from build123d import *

# Parameters (mm, degrees)
SKETCH_1_R                      = 75
SKETCH_1_R_2                    = 50
EXTRUDE_1_DEPTH                 = 50
SKETCH_2_R                      = 525
SKETCH_2_R_2                    = 500
EXTRUDE_2_DEPTH                 = 50
EXTRUDE_4_DEPTH                 = 25
CUT_EXTRUDE_1_DEPTH             = 10
PATTERN_CIRCULAR_1_COUNT        = 5
PATTERN_CIRCULAR_1_COPY_1_DEPTH = 10
PATTERN_CIRCULAR_1_COPY_2_DEPTH = 10
PATTERN_CIRCULAR_1_COPY_3_DEPTH = 10
PATTERN_CIRCULAR_1_COPY_4_DEPTH = 10


with BuildPart() as part:
    # Sketch 1 → Extrude 1 (new body, symmetric)
    with BuildSketch(Plane(origin=(0, 0, 0), x_dir=(1, 0, 0), z_dir=(0, 1, 0))):
        Circle(SKETCH_1_R)
        Circle(SKETCH_1_R_2, mode=Mode.SUBTRACT)
    extrude(amount=EXTRUDE_1_DEPTH, both=True)



with BuildPart() as body_2:
    # Sketch 2 → Extrude 2 (new body, symmetric)
    with BuildSketch(Plane(origin=(0, 0, 0), x_dir=(1, 0, 0), z_dir=(0, 1, 0))):
        Circle(SKETCH_2_R)
        Circle(SKETCH_2_R_2, mode=Mode.SUBTRACT)
    extrude(amount=EXTRUDE_2_DEPTH, both=True)


with BuildPart() as part_1:
    add(part.part)

    add(body_2.part)  # Extrude 4 merges body 2
    # Sketch 3 → Extrude 4 (add, symmetric)
    with BuildSketch(Plane(origin=(0, 0, 0), x_dir=(1, 0, 0), z_dir=(0, 1, 0))):
        with BuildLine():
            Line((487.740991927, -160.966827682), (47.481076098, -15.669952538))
            ThreePointArc((47.481076098, -15.669952538), (45.762156741, -20.145098917), (43.622562007, -24.435058502))
            Line((43.622562007, -24.435058502), (449.989958214, -252.06064129))
            Line((449.989958214, -252.06064129), (487.740991927, -160.966827682))
        make_face()
        with BuildLine():
            ThreePointArc((-0.230551046, -49.999468459), (-5.017843464, -49.747575287), (-9.759008616, -49.038370189))
            Line((-9.759008616, -49.038370189), (-100.669371014, -505.856903799))
            Line((-100.669371014, -505.856903799), (-2.368295015, -513.610733921))
            Line((-2.368295015, -513.610733921), (-0.230551046, -49.999468459))
        make_face()
        with BuildLine():
            ThreePointArc((-47.623564481, -15.231418389), (-48.863354552, -10.600593468), (-49.653961028, -5.872321028))
            Line((-49.653961028, -5.872321028), (-512.207051127, -60.576118701))
            Line((-512.207051127, -60.576118701), (-489.204678742, -156.462062868))
            Line((-489.204678742, -156.462062868), (-47.623564481, -15.231418389))
        make_face()
        with BuildLine():
            ThreePointArc((-29.202430469, 40.585934198), (-25.181370454, 43.196048223), (-20.928826975, 45.409076201))
            Line((-20.928826975, 45.409076201), (-215.89199586, 468.418803535))
            Line((-215.89199586, 468.418803535), (-299.976823903, 416.911861118))
            Line((-299.976823903, 416.911861118), (-29.202430469, 40.585934198))
        make_face()
        with BuildLine():
            ThreePointArc((29.575469897, 40.314905189), (33.300411729, 37.29721945), (36.719234612, 33.936673518))
            Line((36.719234612, 33.936673518), (378.778459787, 350.074860255))
            Line((378.778459787, 350.074860255), (303.808805733, 414.127763353))
            Line((303.808805733, 414.127763353), (29.575469897, 40.314905189))
        make_face()
    extrude(amount=EXTRUDE_4_DEPTH, both=True)

    # Sketch 4 → Cut-Extrude 1 (cut)
    with BuildSketch(Plane.XZ.offset(25)):
        Polygon((-72.052388825, 465.166723777), (-44.040818004, 437.155152956), (-23.032139887, 465.166723777), (-16.029247182, 197.055974487), align=None)
    cut_extrude_1 = extrude(amount=-CUT_EXTRUDE_1_DEPTH, mode=Mode.SUBTRACT)

    # Mirror 1: Cut-Extrude 1 across plane
    add(cut_extrude_1.mirror(Plane.ZX), mode=Mode.SUBTRACT)

    # Pattern Circular 1: Cut-Extrude 1 ×5 about axis
    pattern_circular_1_axis = Axis((0, 0, 0), (0, 1, 0))
    for i in range(1, PATTERN_CIRCULAR_1_COUNT):
        add(cut_extrude_1.rotate(pattern_circular_1_axis, i * 360 / PATTERN_CIRCULAR_1_COUNT), mode=Mode.SUBTRACT)

    # Pattern Circular 1 copy 1 sketch → Pattern Circular 1 copy 1 (cut)
    with BuildSketch(Plane(origin=(0, 25, 0), x_dir=(0.309016994, 0, -0.951056516), z_dir=(0, 1, 0))):
        Polygon((-72.052388825, -465.166723777), (-44.040818004, -437.155152956), (-23.032139887, -465.166723777), (-16.029247182, -197.055974487), align=None)
    extrude(amount=-PATTERN_CIRCULAR_1_COPY_1_DEPTH, mode=Mode.SUBTRACT)

    # Pattern Circular 1 copy 2 sketch → Pattern Circular 1 copy 2 (cut)
    with BuildSketch(Plane(origin=(0, 25, 0), x_dir=(-0.809016994, 0, -0.587785252), z_dir=(0, 1, 0))):
        Polygon((-72.052388825, -465.166723777), (-44.040818004, -437.155152956), (-23.032139887, -465.166723777), (-16.029247182, -197.055974487), align=None)
    extrude(amount=-PATTERN_CIRCULAR_1_COPY_2_DEPTH, mode=Mode.SUBTRACT)

    # Pattern Circular 1 copy 3 sketch → Pattern Circular 1 copy 3 (cut)
    with BuildSketch(Plane(origin=(0, 25, 0), x_dir=(-0.809016994, 0, 0.587785252), z_dir=(0, 1, 0))):
        Polygon((-72.052388825, -465.166723777), (-44.040818004, -437.155152956), (-23.032139887, -465.166723777), (-16.029247182, -197.055974487), align=None)
    extrude(amount=-PATTERN_CIRCULAR_1_COPY_3_DEPTH, mode=Mode.SUBTRACT)

    # Pattern Circular 1 copy 4 sketch → Pattern Circular 1 copy 4 (cut)
    with BuildSketch(Plane(origin=(0, 25, 0), x_dir=(0.309016994, 0, 0.951056516), z_dir=(0, 1, 0))):
        Polygon((-72.052388825, -465.166723777), (-44.040818004, -437.155152956), (-23.032139887, -465.166723777), (-16.029247182, -197.055974487), align=None)
    extrude(amount=-PATTERN_CIRCULAR_1_COPY_4_DEPTH, mode=Mode.SUBTRACT)


solid = part_1.part
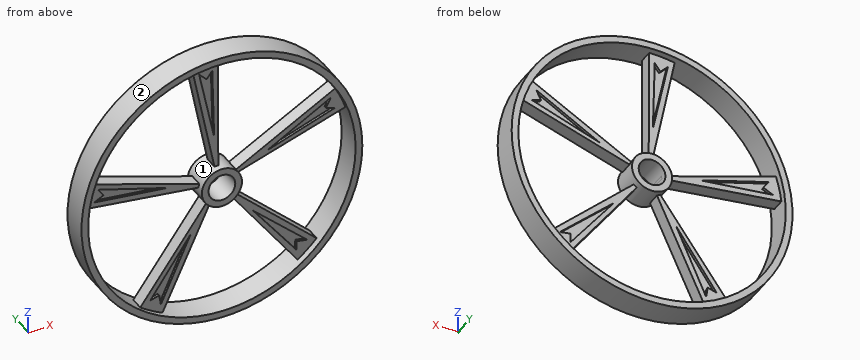
Input: part model. Units: mm. Frame: model coordinates. Face numbers are marked on the shaded views. Coordinates: 2 decimals unless noted, no trailing zeros. Loops run counter-clockwise (first coordinate to the right, second up) from the corner with the lowest first, then second, coordinate; pieces in that order, holes last.
(1) Section C-C on z = -91.5. Return the cut outline in (x, y).
(2) First-contact query: pin 1 Ø5 at (y, z) = (-18, -404) entering from +X; pin 2 Ø1 at (x, y) = (298, -30.5) entering from +Z; pin 3 Ø10 at (x, z) = (-389.5, 75.5) entering from +Y. Flat tips, straight axial feed; report the tip coordinate or a pass-through.
(3) Section A-A on x = 98. Return the cut outline in (y, z), then the cut area to 3 significant figures.
(4) Material intervals for probe 1 along X at (y, z) = (7, 0); probe 2 along X at (y, z) = (-4, -112), sorted ascending.
(5) Section B-B on z = 308.5. Return the cut outline in (x, y).
(6) Pull-direction query (X, two-part tool) for the marked faces 1 and 2; classes: released by +X, released by -X, zero draft, split by the parting line, or undercut.
Data:
1. outline: (-516.96, -50) - (-491.56, -50) - (-491.56, 50) - (-516.96, 50) - close; (-65.84, -25) - (-42.17, -25) - (-42.17, 25) - (-65.84, 25) - close; (67.13, -25) - (99, -25) - (99, 25) - (67.13, 25) - close; (491.56, -50) - (516.96, -50) - (516.96, 50) - (491.56, 50) - close
2. pin 1: stops at x = 338.26
2. pin 2: stops at z = 432.57
2. pin 3: stops at y = 15
3. outline: (-50, -515.77) - (50, -515.77) - (50, -490.3) - (-50, -490.3) - close; (-50, 490.3) - (50, 490.3) - (50, 515.77) - (-50, 515.77) - close; (-25, -133.59) - (25, -133.59) - (25, -90.57) - (-25, -90.57) - close; (-25, 32.34) - (25, 32.34) - (25, 54.89) - (-25, 54.89) - close
3. area: 8,370 mm2
4. probe 1: x = -525 to -500, -75 to -50, 50 to 75, 500 to 525
4. probe 2: x = -512.91 to -487.29, -80.59 to -51.62, 82.16 to 121.18, 487.29 to 512.91
5. outline: (-424.8, -50) - (-393.48, -50) - (-393.48, 50) - (-424.8, 50) - close; (-61.39, -25) - (-39.32, -25) - (-39.32, -15) - (-18.94, -15) - (-18.94, -25) - (-1.42, -25) - (-1.42, 25) - (-18.94, 25) - (-18.94, 15) - (-39.32, 15) - (-39.32, 25) - (-61.39, 25) - close; (393.48, -50) - (424.8, -50) - (424.8, 50) - (393.48, 50) - close
6. face 1: undercut
6. face 2: split by the parting line
